from build123d import *

# Parameters (mm, degrees)
RESSALTO_EXTRUS_O1_DEPTH = 60
CHANFRO1_SIZE            = 20
ESBO_O2_R                = 6
CORTE_EXTRUS_O1_DEPTH    = 163.7


with BuildPart() as part:
    # Esboço1 → Ressalto-extrusão1 (new body, symmetric)
    with BuildSketch(Plane.XY):
        Polygon((-100, 0), (100, 0), (100, 12.7), (62.7, 12.7), (62.7, 100), (50, 100), (50, 20), (-50, 20), (-50, 100), (-62.7, 100), (-62.7, 12.7), (-100, 12.7), align=None)
    extrude(amount=RESSALTO_EXTRUS_O1_DEPTH, both=True)

    # Chanfro1
    chanfro1_edges = [part.edges().sort_by_distance(p)[0] for p in [
        (-56.35, 100, -60),
        (56.35, 100, 60),
        (56.35, 100, -60),
        (-56.35, 100, 60),
    ]]
    chamfer(chanfro1_edges, length=CHANFRO1_SIZE)

    # Esboço2 → Corte-extrusão1 (cut, through all)
    with BuildSketch(Plane(origin=(62.7, 0, 0), x_dir=(0, 0, -1), z_dir=(1, 0, 0))):
        with Locations((-35, 80)):
            Circle(ESBO_O2_R)
        with Locations((35, 80)):
            Circle(ESBO_O2_R)
    extrude(amount=-CORTE_EXTRUS_O1_DEPTH, mode=Mode.SUBTRACT)


solid = part.part
Check sheet for the modelled part. Datum: model origin and axes. Units: mm. A direction names the side the tool comes from. Round coordinates to 2 decimals unless told otherwise and drop trailing zeros. Order: outer loops, then holes, each group sorted by start corner. A loop starts at its lowest first (then second) coordinate and runs counter-clockwise, first axis right, second up.
(1) Access from +Z, -Z, +X, -X, +Y, -Y to the whole of each face (thin tool, end or side, straight path). Record for faces 1 (the flat face through (-50, 59, 1)), 2 (the flat face through (62.7, 56, 1)), 3 (the flat face through (-81, 12.7, 1)).
(2) Draft check along Y on faces 4 (the cylindrical face through (-56.26, 84.06, 39.42)), 5 (the flat face through (56, 90, -50)), 6 (the flat face through (0, 14, 60)). Enter one of: pulls with the +Y half, pulls with the -Y half, needs draft (parallel to the pull), parting line crosses it, or undercut.
(3) Cross-section at B-B, the plane z = -35. Enter the section's corners in (x, y), and give its area (3 significant figures).
(4) Scan lines: probe 1 along X at (y, z) = (87.5, -32.5); probe 2 along Y at (x, z) = (-54, 35); probe 3 along Y at (x, z) = (-68.5, -37). Record each from-to range of solid material in increasing order.
(5) Cross-section at A-A, the plane y = 57.5. Enter the section's corners in (x, z).
(6) Go/stop test with flat-tipped pins: P1, Ø24, axis at y = 44, z = -21, coming from the -X side; P2, Ø1.5, axis at x = 0.5, z = 36.5, coming from the +Y side; P3, Ø9.5, axis at y = 80, z = -35, coming from the +X side; P4, Ø5, axis at x = 74.5, z = -15, coming from the +Y side. Record where each tip stops, or that it passes through.
(7) Cross-section at D-D, the plane x = -85. Enter the section's corners in (y, z), and give its area (3 significant figures).
(8) Cross-section at C-C, the plane z = 47. Enter the section's corners in (x, y), and give its area (3 significant figures).
Check sheet entries:
1. face 1: +Z, -Z, +Y
1. face 2: +Z, -Z, +X, +Y
1. face 3: +Z, -Z, -X, +Y
2. face 4: undercut
2. face 5: pulls with the +Y half
2. face 6: needs draft
3. outline: (-100, 0) - (100, 0) - (100, 12.7) - (62.7, 12.7) - (62.7, 74) - (50, 74) - (50, 20) - (-50, 20) - (-50, 74) - (-62.7, 74) - (-62.7, 12.7) - (-100, 12.7) - close; (-62.7, 86) - (-50, 86) - (-50, 100) - (-62.7, 100) - close; (50, 86) - (62.7, 86) - (62.7, 100) - (50, 100) - close
3. area: 5,180 mm2
4. probe 1: x = -62.7 to -50, 50 to 62.7
4. probe 2: y = 0 to 74, 86 to 100
4. probe 3: y = 0 to 12.7
5. outline: (-62.7, -60) - (-50, -60) - (-50, 60) - (-62.7, 60) - close; (50, -60) - (62.7, -60) - (62.7, 60) - (50, 60) - close
6. P1: stops at x = -62.7
6. P2: stops at y = 20
6. P3: passes through
6. P4: stops at y = 12.7
7. outline: (0, -60) - (12.7, -60) - (12.7, 60) - (0, 60) - close
7. area: 1,520 mm2
8. outline: (-100, 0) - (100, 0) - (100, 12.7) - (62.7, 12.7) - (62.7, 93) - (50, 93) - (50, 20) - (-50, 20) - (-50, 93) - (-62.7, 93) - (-62.7, 12.7) - (-100, 12.7) - close
8. area: 5,310 mm2
